Read the model definition and answer for the solid it produces. Units are mm, in the model's axes. Face numbers are marked on the shaded views. Coordinates: 2 decimals unless noted, no trailing zeros. Loops run counter-clockwise (first coordinate to the right, second up) from the corner with the lowest first, then second, coordinate; pieces in that order, holes last. Notation, with made-up numbers: M -4,-28.5 L 40,-28.5 A29 cw 40,-6.5 Z; hole C -30,-22 d5. An arc over 180 degrees is marked long. Put each result on its own line as item: value.
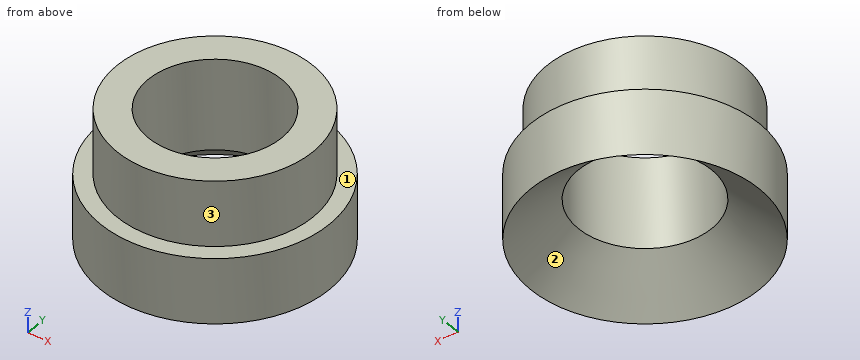
from build123d import *

# Parameters (mm, degrees)
SKETCH1_R                                           = 5.55625
BOSS_EXTRUDE1_DEPTH                                 = 3.175
SKETCH2_R                                           = 4.7625
BOSS_EXTRUDE2_DEPTH                                 = 3.175
CSK_FOR_1_4_FLAT_HEAD_MACHINE_SCREW_100_D           = 6.477
CSK_FOR_1_4_FLAT_HEAD_MACHINE_SCREW_100_CSINK_D     = 11.1125
CSK_FOR_1_4_FLAT_HEAD_MACHINE_SCREW_100_CSINK_ANGLE = 100


with BuildPart() as part:
    # Sketch1 → Boss-Extrude1 (new body)
    with BuildSketch(Plane.XY):
        Circle(SKETCH1_R)
    extrude(amount=BOSS_EXTRUDE1_DEPTH)

    # Sketch2 → Boss-Extrude2 (add)
    with BuildSketch(Plane.XY.offset(3.175)):
        Circle(SKETCH2_R)
    extrude(amount=BOSS_EXTRUDE2_DEPTH)

    # CSK for 1/4 Flat Head Machine Screw (100)1 (through all)
    with Locations(Plane(origin=(0, 0, 0), x_dir=(-1, 0, 0), z_dir=(0, 0, -1))):
        with Locations((0, 0)):
            CounterSinkHole(CSK_FOR_1_4_FLAT_HEAD_MACHINE_SCREW_100_D / 2, CSK_FOR_1_4_FLAT_HEAD_MACHINE_SCREW_100_CSINK_D / 2, counter_sink_angle=CSK_FOR_1_4_FLAT_HEAD_MACHINE_SCREW_100_CSINK_ANGLE)


solid = part.part
1) Straight lines are drawn through the part: line 1 (Y direction, x = 0, z = 4.35); line 2 (Y direction, x = 0, z = 3.05); line 3 (X direction, y = -0.5, z = 3.25). For each, find the intervals that lie inside material, in ascending order. Write a range as [from, to].
Answer list:
line 1: y = [-4.76, -3.24], [3.24, 4.76]
line 2: y = [-5.56, -3.24], [3.24, 5.56]
line 3: x = [-4.74, -3.2], [3.2, 4.74]
2) Find section D-D, the plane z = 3. Write down the section's boundary in (x, y).
Answer list:
outline: C 0,0 d11.11; hole C 0,0 d6.48
3) Find section C-C, the plane z = 5.75. Write down the section's boundary in (x, y) (1 decimal), plus the area to 3 significant figures.
Answer list:
outline: C 0,0 d9.5; hole C 0,0 d6.5
area: 38.3 mm^2
4) Determine the mould class of the marked faces 1, 2 and 3 for opening direction Y: released by +Y, released by -Y, zero draft, split by the parting line, or undercut.
Answer list:
face 1: zero draft
face 2: undercut
face 3: split by the parting line
5) Given pin 1 Ø1.5 at (x, y) = (-1.5, 1) entering from -Z; pin 2 Ø3 at (x, z) = (1.5, 4) entering from +Y; pin 3 Ø5.5 at (x, y) = (1, 0) entering from +Z, each flat-ended and moving along its own axis, determine where each tip first touches the part or whether it passes through.
Answer list:
pin 1: passes through
pin 2: stops at y = 5.55
pin 3: stops at z = 6.35
